from build123d import *

# Parameters (mm, degrees)
F0_W     = 20
F0_H     = 5
F1_DEPTH = 8
F2_R     = 2
F3_DEPTH = 2
F4_SIZE  = 0.2


with BuildPart() as f1:
    # F0 (on Top) → F1 (new body)
    with BuildSketch(Plane.XY):
        with Locations((-10, 2.5)):
            Rectangle(F0_W, F0_H)
    extrude(amount=F1_DEPTH)

    # F2 (on face) → F3 (join)
    with BuildSketch(Plane.XY.offset(8)):
        with Locations((-17, 2.409057)):
            Circle(F2_R)
        with Locations((-10, 2.63126)):
            Circle(F2_R)
        with Locations((-3, 2.747634)):
            Circle(F2_R)
    extrude(amount=F3_DEPTH)

    # F4
    f4_edges = [f1.edges().sort_by_distance(p)[0] for p in [
        (-19, 2.409057, 10),
        (-12, 2.63126, 10),
        (-5, 2.747634, 10),
    ]]
    chamfer(f4_edges, length=F4_SIZE)


solid = f1.part
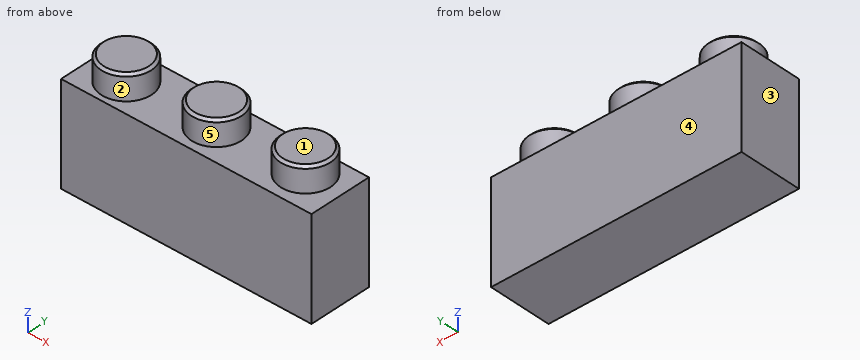
Design review of the part built by this model. Coordinates are the model's own, in mm. Face numbers are marked on the shaded views. A direction names the side the tool comes from. Coordinates: 2 decimals unless noted, no trailing zeros. Order: outer loops, then holes, each group sorted by start corner. A loop starts at its lowest first (then second) coordinate and runs counter-clockwise, first axis right, second up.
Item 1: Take a section at B-B, the plane z = 8.75. Write out the cut boundary in (x, y), then the cut area to 3 significant figures.
Item 2: For the marked faces 1 and 2, list the 3-axis set-ups (+Z, -Z, +X, -X, +Y, -Y) from which the entire face can be reached by the end or side of a thin tool; tool diameter is ignored.
Item 3: The part is to be moulded in two halves that separate along X. For the marked faces 3, 4 and 5, say which applies: pulls with the +X half, pulls with the -X half, needs draft (parallel to the pull), parting line crosses it, or undercut.
Item 4: Take a section at C-C, the plane x = -7.25. Write out the cut boundary in (y, z), then the cut area to 3 significant figures.
Item 5: Take a section at A-A, the plane x = -10. Write out the cut boundary in (y, z), then the cut area to 3 significant figures.
Item 6: For line 1 (X direction, y = 3.1, z = 9); line 2 (Z direction, x = -14, y = 1.75); line 3 (X direction, y = 3.8, z = 8.25), list the stretches that pass through material, from the lowest coordinate up.
The answers:
1. outline: circle Ø4 at (-17, 2.41); circle Ø4 at (-10, 2.63); circle Ø4 at (-3, 2.75)
1. area: 37.7 mm2
2. face 1: +Z, +X, -X, +Y, -Y
2. face 2: +Z
3. face 3: pulls with the -X half
3. face 4: needs draft
3. face 5: undercut
4. outline: (0, 0) - (5, 0) - (5, 8) - (0, 8) - close
4. area: 40.0 mm2
5. outline: (0, 0) - (5, 0) - (5, 8) - (4.63, 8) - (4.63, 9.8) - (4.43, 10) - (0.83, 10) - (0.63, 9.8) - (0.63, 8) - (0, 8) - close
5. area: 48.0 mm2
6. line 1: x = -18.88 to -15.12, -11.94 to -8.06, -4.97 to -1.03
6. line 2: z = 0 to 8
6. line 3: x = -18.44 to -15.56, -11.62 to -8.38, -4.7 to -1.3
